Job drawing, mm, ordinate dimensions from the low corner. One solid piece. A direction names the side the tool comes from. Give positions to 0.01 mm unless a question says otherwise; leave off trailing zeros. Order: outer loops, then holes, each group sorted by start corner. A loop starts at its lowest first (then second) coordinate and runs counter-clockwise, first axis right, second up.
Item 1: Which spindle directions (+Z, -Z, +X, -X, +Y, -Y) get a long thin tool onto all of the face, cutting with end or side? Do the marked faces 5 and 6. Say none if no direction does.
Item 2: Band-saw the part on C-C on y = 0.3. Give the cut face in (x, z).
Item 3: Wall check: L1, parallel to Z at x = 10, y = 0.8; L2, parallel to Y at x = 12.75, z = 3; L3, parallel to Z at x = 17.25, y = 1.3. Give the ranges that are in metal, low to high.
Item 4: Band-saw the part on A-A on x = 10. Give the cut face in (y, z).
Item 5: Band-saw the part on B-B on z = 10. Give the cut face in (x, y), plus the area to 3 significant figures.
Item 6: Flat gauge pins, fed straight in: P1, Ø6, axis at x = 6.5, z = 9, coming from the +Y side; P2, Ø1.5, axis at y = 1.5, z = 2.5, coming from the +X side; P3, Ø2.5, axis at x = 10, z = 18, coming from the +Y side; P4, Ø1.5, axis at x = 4, y = 2, coming from the -Z side. Where does each tip first touch, or does it go through?
Item 7: Two-plate mould, pull along X, no slides. Class the marked faces 1, 2, 3 and 4: released by +X, released by -X, zero draft, split by the parting line, or undercut.
Item 8: Band-saw the part on D-D on x = 2. Give the cut face in (y, z).
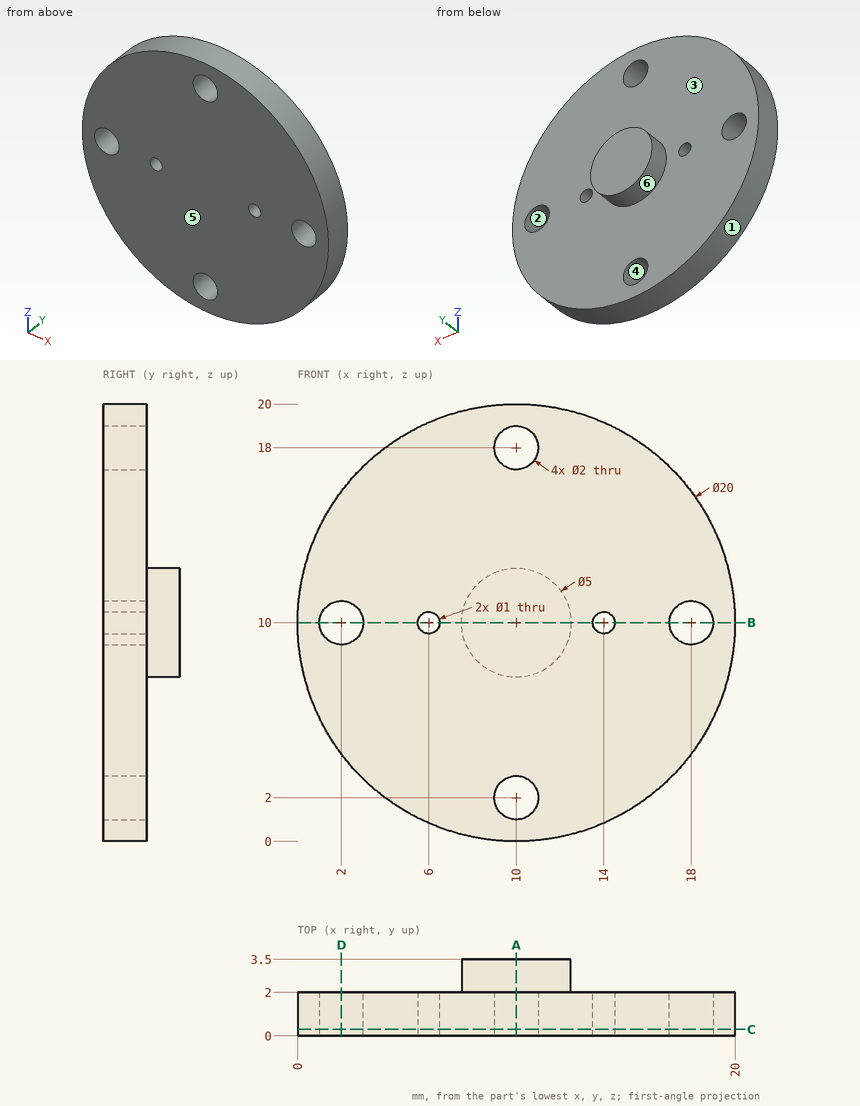
The answers:
1. face 5: +Z, -Z, +X, -X, -Y
1. face 6: +Y
2. outline: circle Ø20 at (10, 10); hole circle Ø2 at (2, 10); hole circle Ø1 at (6, 10); hole circle Ø2 at (10, 2); hole circle Ø2 at (10, 18); hole circle Ø1 at (14, 10); hole circle Ø2 at (18, 10)
3. L1: z = 0 to 1, 3 to 17, 19 to 20
3. L2: y = 0 to 2
3. L3: z = 3.11 to 9.34, 10.66 to 16.89
4. outline: (0, 0) - (2, 0) - (2, 1) - (0, 1) - close; (0, 3) - (2, 3) - (2, 7.5) - (3.5, 7.5) - (3.5, 12.5) - (2, 12.5) - (2, 17) - (0, 17) - close; (0, 19) - (2, 19) - (2, 20) - (0, 20) - close
5. outline: (0, 0) - (1, 0) - (1, 2) - (0, 2) - close; (3, 0) - (5.5, 0) - (5.5, 2) - (3, 2) - close; (6.5, 0) - (13.5, 0) - (13.5, 2) - (12.5, 2) - (12.5, 3.5) - (7.5, 3.5) - (7.5, 2) - (6.5, 2) - close; (14.5, 0) - (17, 0) - (17, 2) - (14.5, 2) - close; (19, 0) - (20, 0) - (20, 2) - (19, 2) - close
5. area: 35.5 mm2
6. P1: stops at y = 3.5
6. P2: stops at x = 17.38
6. P3: stops at y = 2
6. P4: stops at z = 1.49
7. face 1: split by the parting line
7. face 2: undercut
7. face 3: zero draft
7. face 4: undercut
8. outline: (0, 4) - (2, 4) - (2, 9) - (0, 9) - close; (0, 11) - (2, 11) - (2, 16) - (0, 16) - close
